Here's how the part is built. I have some questions about the finished solid (model axes, mm). A direction names the side the tool comes from. Coordinates: 2 decimals unless noted, no trailing zeros. Order: outer loops, then holes, each group sorted by start corner. A loop starts at its lowest first (then second) coordinate and runs counter-clockwise, first axis right, second up. Notation, with made-up numbers: (42.5, -31) - (64.5, -31) arc R23 cw to (64.5, 1) - close; hole circle Ø3 at (85.5, 47). An arc over 180 degrees is marked (long way). Use CSV: the item, a comma, the result in double quotes. Start each with the question number.
from build123d import *

# Parameters (mm, degrees)
ESQUISSE1_R             = 3
ESQUISSE1_W             = 51
ESQUISSE1_H             = 19.5
BOSS_EXTRU_1_DEPTH      = 2
BOSS_EXTRU_2_DEPTH      = 13
ESQUISSE3_W             = 2
ESQUISSE3_H             = 8.661779492
ESQUISSE3_H_2           = 8.71590367
ESQUISSE3_H_3           = 8.44528278
ESQUISSE3_H_4           = 8.493191711
ENL_V_MAT_EXTRU_1_DEPTH = 5


with BuildPart() as part:
    # Esquisse1 → Boss.-Extru.1 (new body)
    with BuildSketch(Plane.XY):
        with BuildLine():
            Line((-5, 30), (56, 30))
            ThreePointArc((56, 30), (63.071067812, 27.071067812), (66, 20))
            Line((66, 20), (66, -30))
            ThreePointArc((66, -30), (63.071067812, -37.071067812), (56, -40))
            Line((56, -40), (-5, -40))
            ThreePointArc((-5, -40), (-12.071067812, -37.071067812), (-15, -30))
            Line((-15, -30), (-15, 20))
            ThreePointArc((-15, 20), (-12.071067812, 27.071067812), (-5, 30))
        make_face()
        with Locations((0, -16)):
            Circle(ESQUISSE1_R, mode=Mode.SUBTRACT)
        with Locations((25.5, -16)):
            Circle(ESQUISSE1_R, mode=Mode.SUBTRACT)
        with Locations((51, -16)):
            Circle(ESQUISSE1_R, mode=Mode.SUBTRACT)
        with Locations((25.5, 9.75)):
            Rectangle(ESQUISSE1_W, ESQUISSE1_H, mode=Mode.SUBTRACT)
    extrude(amount=BOSS_EXTRU_1_DEPTH)

    # Esquisse2 → Boss.-Extru.2 (add)
    with BuildSketch(Plane.XY.offset(2)):
        with BuildLine():
            Line((-5, 30), (56, 30))
            ThreePointArc((56, 30), (63.071067812, 27.071067812), (66, 20))
            Line((66, 20), (66, -30))
            ThreePointArc((66, -30), (63.071067812, -37.071067812), (56, -40))
            Line((56, -40), (-5, -40))
            ThreePointArc((-5, -40), (-12.071067812, -37.071067812), (-15, -30))
            Line((-15, -30), (-15, 20))
            ThreePointArc((-15, 20), (-12.071067812, 27.071067812), (-5, 30))
        make_face()
        with BuildLine():
            Line((-13.5, 18.5), (-13.5, -28.5))
            ThreePointArc((-13.5, -28.5), (-10.571067812, -35.571067812), (-3.5, -38.5))
            Line((-3.5, -38.5), (54.5, -38.5))
            ThreePointArc((54.5, -38.5), (61.571067812, -35.571067812), (64.5, -28.5))
            Line((64.5, -28.5), (64.5, 18.5))
            ThreePointArc((64.5, 18.5), (61.571067812, 25.571067812), (54.5, 28.5))
            Line((54.5, 28.5), (-3.5, 28.5))
            ThreePointArc((-3.5, 28.5), (-10.571067812, 25.571067812), (-13.5, 18.5))
        make_face(mode=Mode.SUBTRACT)
    extrude(amount=BOSS_EXTRU_2_DEPTH)

    # Esquisse3 → Enlèv. mat.-Extru.1 (cut)
    with BuildSketch(Plane(origin=(0, 0, 0), x_dir=(-1, 0, 0), z_dir=(0, 0, -1))):
        with Locations((-25.5, 29.330889746)):
            Rectangle(ESQUISSE3_W, ESQUISSE3_H)
        with Locations((-31.5, 29.357951835)):
            Rectangle(ESQUISSE3_W, ESQUISSE3_H_2)
        with Locations((-19.5, 29.22264139)):
            Rectangle(ESQUISSE3_W, ESQUISSE3_H_3)
        with Locations((-25.5, -39.246595856)):
            Rectangle(ESQUISSE3_W, ESQUISSE3_H_4)
        with Locations((-31.5, -39.246595856)):
            Rectangle(ESQUISSE3_W, ESQUISSE3_H_4)
        with Locations((-19.5, -39.246595856)):
            Rectangle(ESQUISSE3_W, ESQUISSE3_H_4)
    extrude(amount=-ENL_V_MAT_EXTRU_1_DEPTH, mode=Mode.SUBTRACT)


solid = part.part
Item 1: Suppose I cut it at A-A on x = 12. Write out the boundary of the cut face in (y, z).
Item 2: For faces 4 (the flat face through (20, -35, 1)), 5 (the flat face through (26, -12, 2)), 6 (the flat face through (20.5, -38, 1)), 7 (the flat face through (51, 10, 1)), which set-ups out of +Z, -Z, +X, -X, +Y, -Y let a thin tool reach every point of the face, with its end or its side?
Item 3: For pin 1 Ø2.5 at (y, z) = (27.5, 1.5) entering from -X; pin 2 Ø3 at (x, y) = (36.5, -4.5) entering from +Z; pin 3 Ø1.5 at (y, z) = (28.5, 3) entering from +X, each with a flat end and sliding along its axis, tell me the tip position at first contact or that it passes through.
Item 4: Suppose I cut it at C-C on y = 16. Write out the boundary of the cut face in (x, z).
Item 5: Suppose I cut it at D-D on z = 12.5. Write out the boundary of the cut face in (x, y).
Item 6: We'd pull the mould along X, two halves only. Please class faces 1 (the flat face through (65, -5, 15)), 2 (the flat face through (66, -5, 7)), 3 (the flat face through (-13.5, -5, 8)): released by +X, released by -X, zero draft, split by the parting line, or undercut.
Item 7: Suppose I cut it at B-B on y = -16. Write out the boundary of the cut face in (x, z), then the cut area to 3 significant figures.
Item 8: Please list where these lines run through material, in increasing order: line 1 along Y through (x, z) = (25.5, 1.1); line 2 along X through (y, z) = (-9.5, 4); line 3 along Y through (x, z) = (12.5, 6.25). Write a range as from..to.
Here are the results:
1,outline,"(-40, 0) - (0, 0) - (0, 2) - (-38.5, 2) - (-38.5, 15) - (-40, 15) - close; (19.5, 0) - (30, 0) - (30, 15) - (28.5, 15) - (28.5, 2) - (19.5, 2) - close"
2,face 4,"+Z, -Z, -Y"
2,face 5,"+Z"
2,face 6,"-Z, -Y"
2,face 7,"+Z, -Z"
3,pin 1,"x = -12.81"
3,pin 2,"z = 2"
3,pin 3,"x = 62.32"
4,outline,"(-15, 0) - (0, 0) - (0, 2) - (-13.5, 2) - (-13.5, 15) - (-15, 15) - close; (51, 0) - (66, 0) - (66, 15) - (64.5, 15) - (64.5, 2) - (51, 2) - close"
5,outline,"(-15, -30) arc R10 ccw to (-5, -40) - (56, -40) arc R10 ccw to (66, -30) - (66, 20) arc R10 ccw to (56, 30) - (-5, 30) arc R10 ccw to (-15, 20) - close; hole (-13.5, -28.5) arc R10 ccw to (-3.5, -38.5) - (54.5, -38.5) arc R10 ccw to (64.5, -28.5) - (64.5, 18.5) arc R10 ccw to (54.5, 28.5) - (-3.5, 28.5) arc R10 ccw to (-13.5, 18.5) - close"
6,face 1,"zero draft"
6,face 2,"released by +X"
6,face 3,"undercut"
7,outline,"(-15, 0) - (-3, 0) - (-3, 2) - (-13.5, 2) - (-13.5, 15) - (-15, 15) - close; (3, 0) - (22.5, 0) - (22.5, 2) - (3, 2) - close; (28.5, 0) - (48, 0) - (48, 2) - (28.5, 2) - close; (54, 0) - (66, 0) - (66, 15) - (64.5, 15) - (64.5, 2) - (54, 2) - close"
7,area,"165 mm^2"
8,line 1,"-35..-19, -13..0, 19.5..25"
8,line 2,"-15..-13.5, 64.5..66"
8,line 3,"-40..-38.5, 28.5..30"
